Can you work these out from the model? Positions are in its coordinate system, mm. Face numbers are marked on the shaded views. A direction names the side the tool comes from. Round coordinates to 2 decimals unless told otherwise and drop trailing zeros. Write each loop counter-clockwise with the first axis right and the second up, starting at its lowest first coordinate (ties: lowest second). Pieces come first, ordered by that corner, then holes. Notation, with made-up numbers: (8, 59) -> (43, 59) arc R21 ccw to (43, 68) -> close; hole circle Ø10 at (84, -6). An arc over 180 degrees is marked (long way). Write item = value, one per line. Start each with the question number.
1) Imagine slicing it at C-C, the plane y = -0.5. State how many separate pieces and enclosed holes the cut face has, then the cut area to 3 significant figures.
2) If I drill on line 1 (X direction, y = -1.2, z = -23); line 2 (Z direction, x = -23.75, y = 4); line 3 (Z direction, x = 15, y = -6), over which ranges is the centre line in solid material (lowest first)?
3) Thinking about a two-plate mould opening in X: for the marked faces 1, 2 and 3, which applies, +X half, -X half, draft (parallel to the pull), parting line (faces both ways), or undercut?
4) I'm going to push flat-ended pins straight in: pin 1 (0.6 mm diameter, centred on x = 8, z = -12.5, fed in from -Y); pin 2 (2 mm diameter, centred on x = 46, z = -9, fed in from +Y); pin 3 (0.6 mm diameter, centred on x = 4, z = -22.5, fed in from +Y). Where does each tip first touch, or does it pass through?
5) Imagine slicing it at A-A, the plane x = -50. Please give me the cut outline in (y, z), then the cut area to 3 significant figures.
6) Imagine slicing it at D-D, the plane x = -23.75. Please give me the cut outline in (y, z).
7) For the marked faces 4, 5, 6 and 7, which set-ups out of +Z, -Z, +X, -X, +Y, -Y let a thin tool reach every point of the face, with its end or its side?
8) Imagine slicing it at B-B, the plane z = -16. Please give me the cut outline in (x, y).
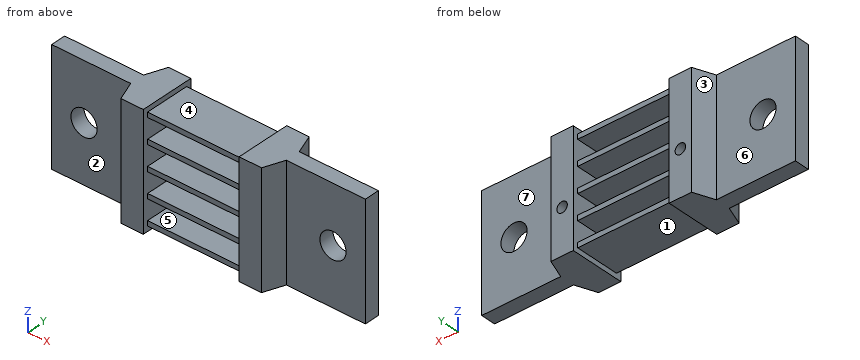
from build123d import *

# Parameters (mm, degrees)
BOSS_EXTRUDE1_DEPTH        = 3
BOSS_EXTRUDE1_DEPTH_BACK   = 3
SKETCH1_W                  = 31.75
SKETCH1_H                  = 46
SKETCH1_R                  = 5.25
BOSS_EXTRUDE1_2_DEPTH      = 3
BOSS_EXTRUDE1_2_DEPTH_BACK = 3
BOSS_EXTRUDE2_DEPTH        = 11
BOSS_EXTRUDE2_DEPTH_BACK   = 11
SKETCH2_W                  = 9
SKETCH2_H                  = 46
BOSS_EXTRUDE2_2_DEPTH      = 11
BOSS_EXTRUDE2_2_DEPTH_BACK = 11
BOSS_EXTRUDE3_DEPTH        = 46
M5X0_8_TAPPED_HOLE1_D      = 4.2
M5X0_8_TAPPED_HOLE1_DEPTH  = 10
BOSS_EXTRUDE4_DEPTH        = 9
BOSS_EXTRUDE4_DEPTH_BACK   = 9
SKETCH6_W                  = 38.5
SKETCH6_H                  = 2


with BuildPart() as part:
    # Sketch1 → Boss-Extrude1 (new, two sides: drawn at the far end of the back side and taken through both)
    with BuildSketch(Plane(origin=(0, 0, 0), x_dir=(1, 0, 0), z_dir=(0, 1, 0)).offset(-BOSS_EXTRUDE1_DEPTH_BACK)):
        with Locations((-47.125, 23)):
            Rectangle(SKETCH1_W, SKETCH1_H)
        with Locations(Location((-50, 23, 0), (0, 0, 270))):
            Circle(SKETCH1_R, mode=Mode.SUBTRACT)
    extrude(amount=BOSS_EXTRUDE1_DEPTH + BOSS_EXTRUDE1_DEPTH_BACK)



with BuildPart() as body_2:
    # Sketch1 → Boss-Extrude1 2 (new, two sides: drawn at the far end of the back side and taken through both)
    with BuildSketch(Plane(origin=(0, 0, 0), x_dir=(1, 0, 0), z_dir=(0, 1, 0)).offset(-BOSS_EXTRUDE1_2_DEPTH_BACK)):
        with Locations((47.125, 23)):
            Rectangle(SKETCH1_W, SKETCH1_H)
        with Locations(Location((50, 23, 0), (0, 0, 270))):
            Circle(SKETCH1_R, mode=Mode.SUBTRACT)
    extrude(amount=BOSS_EXTRUDE1_2_DEPTH + BOSS_EXTRUDE1_2_DEPTH_BACK)


with BuildPart() as body_3:
    # Sketch2 → Boss-Extrude2 (new, two sides: drawn at the far end of the back side and taken through both)
    with BuildSketch(Plane(origin=(0, 0, 0), x_dir=(1, 0, 0), z_dir=(0, 1, 0)).offset(-BOSS_EXTRUDE2_DEPTH_BACK)):
        with Locations((23.75, 23)):
            Rectangle(SKETCH2_W, SKETCH2_H)
    extrude(amount=BOSS_EXTRUDE2_DEPTH + BOSS_EXTRUDE2_DEPTH_BACK)


with BuildPart() as body_4:
    # Sketch2 → Boss-Extrude2 2 (new, two sides: drawn at the far end of the back side and taken through both)
    with BuildSketch(Plane(origin=(0, 0, 0), x_dir=(1, 0, 0), z_dir=(0, 1, 0)).offset(-BOSS_EXTRUDE2_2_DEPTH_BACK)):
        with Locations((-23.75, 23)):
            Rectangle(SKETCH2_W, SKETCH2_H)
    extrude(amount=BOSS_EXTRUDE2_2_DEPTH + BOSS_EXTRUDE2_2_DEPTH_BACK)


with BuildPart() as part_1:
    add(part.part)

    add(body_2.part)  # Boss-Extrude3 merges body 2

    add(body_3.part)  # Boss-Extrude3 merges body 3

    add(body_4.part)  # Boss-Extrude3 merges body 4
    # Sketch3 → Boss-Extrude3 (add, through all)
    with BuildSketch(Plane.XY):
        Polygon((28.25, 11), (31.25, 3), (31.25, -3), (28.25, -11), align=None)
        Polygon((-31.25, 3), (-31.25, -3), (-28.25, -11), (-28.25, 11), align=None)
    extrude(amount=-BOSS_EXTRUDE3_DEPTH)

    # M5x0.8 Tapped Hole1
    with Locations(Plane(origin=(0, 11, 0), x_dir=(1, 0, 0), z_dir=(0, 1, 0))):
        with Locations((-23.75, 28), (23.75, 28)):
            Hole(M5X0_8_TAPPED_HOLE1_D / 2, depth=M5X0_8_TAPPED_HOLE1_DEPTH)

    # Sketch6 → Boss-Extrude4 (add, two sides: drawn at the far end of the back side and taken through both)
    with BuildSketch(Plane(origin=(0, 0, 0), x_dir=(1, 0, 0), z_dir=(0, 1, 0)).offset(-BOSS_EXTRUDE4_DEPTH_BACK)):
        with Locations((0, 2.975890667)):
            Rectangle(SKETCH6_W, SKETCH6_H)
        with Locations((0, 12.975890667)):
            Rectangle(SKETCH6_W, SKETCH6_H)
        with Locations((0, 22.975890667)):
            Rectangle(SKETCH6_W, SKETCH6_H)
        with Locations((0, 32.975890667)):
            Rectangle(SKETCH6_W, SKETCH6_H)
        with Locations((0, 42.975890667)):
            Rectangle(SKETCH6_W, SKETCH6_H)
    extrude(amount=BOSS_EXTRUDE4_DEPTH + BOSS_EXTRUDE4_DEPTH_BACK)


solid = part_1.part
Reported:
q1.separate_pieces = 1
q1.enclosed_holes = 6
q1.area = 4,240 mm²
q2.line_1 = -63 to -55.25, -44.75 to 44.75, 55.25 to 63
q2.line_2 = -46 to -30.1, -25.9 to 0
q2.line_3 = -43.98 to -41.98, -33.98 to -31.98, -23.98 to -21.98, -13.98 to -11.98, -3.98 to -1.98
q3.face_1 = undercut
q3.face_2 = draft
q3.face_3 = -X half
q4.pin_1 = -9
q4.pin_2 = 3
q4.pin_3 = 9
q5.outline = (-3, -46) -> (3, -46) -> (3, -28.25) -> (-3, -28.25) -> close; (-3, -17.75) -> (3, -17.75) -> (3, 0) -> (-3, 0) -> close
q5.area = 213 mm²
q6.outline = (-11, -46) -> (11, -46) -> (11, -30.1) -> (1, -30.1) -> (1, -25.9) -> (11, -25.9) -> (11, 0) -> (-11, 0) -> close
q7.face_4 = +Z, +Y, -Y
q7.face_5 = +Y, -Y
q7.face_6 = +Z, -Z, -X, +Y
q7.face_7 = +Z, -Z, +X, +Y
q8.outline = (-63, -3) -> (-31.25, -3) -> (-28.25, -11) -> (-19.25, -11) -> (-19.25, 11) -> (-28.25, 11) -> (-31.25, 3) -> (-63, 3) -> close; (19.25, -11) -> (28.25, -11) -> (31.25, -3) -> (63, -3) -> (63, 3) -> (31.25, 3) -> (28.25, 11) -> (19.25, 11) -> close
